Part print with two shaded views. Sizes in mm from the minimum x, y, z corner. Give positions to 0.01 mm unless a question says otherwise; leave off trailing zeros. Order: outer loops, then holes, each group sorted by start corner. A loop starts at its lowest first (then second) coordinate and runs counter-clockwise, first axis right, second up. Notation, with made-up numbers: M -21,57.25 L 2,57.25 A15 cw 2,75.25 Z; hole C 45,48.5 d2. An arc over 180 degrees is marked long. Return JSON: item names as keys, results as strings.
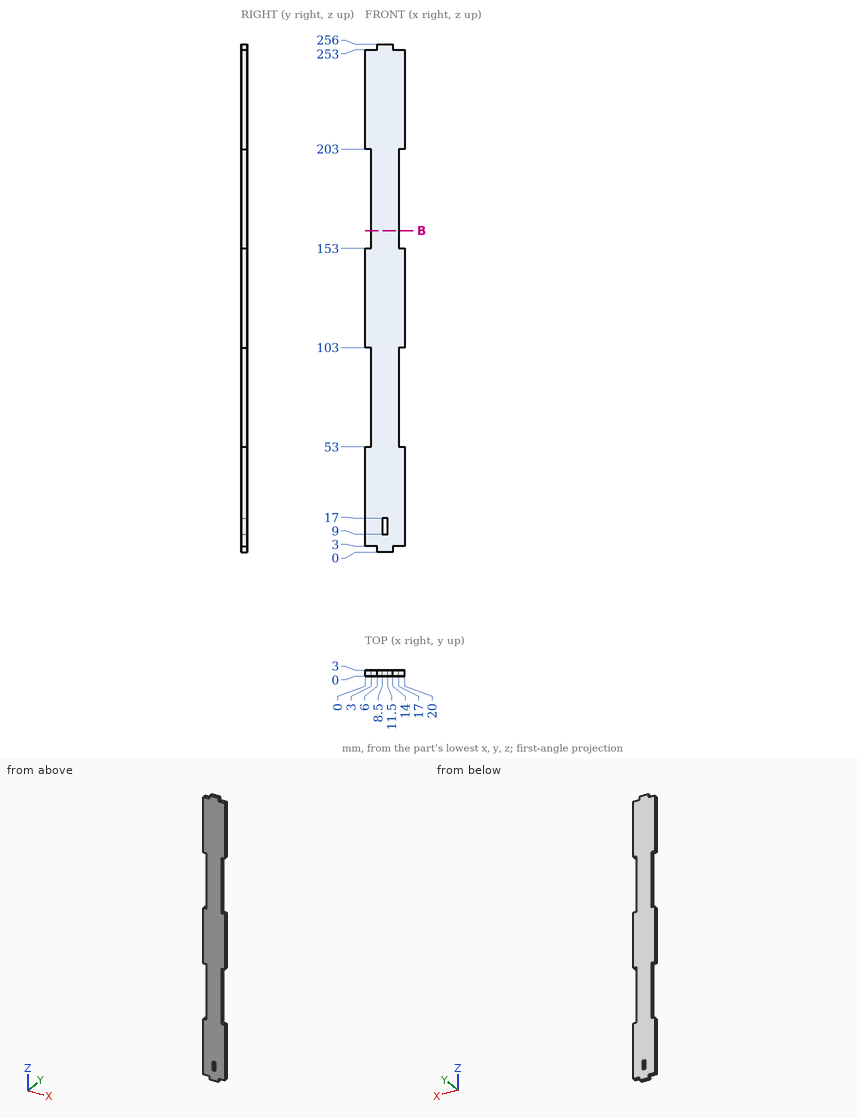
Q1. Band-saw the part on B-B (z = 162). Give the cut face in (x, y).
Established:
{"outline": "M 3,0 L 17,0 L 17,3 L 3,3 Z"}
Q2. Pin check, flat tips, straight feed: pin 1 (0.9 mm diameter, centred on x = 19, y = 1.5, fed in from -Z); pin 2 (1.5 mm diameter, centred on y = 2, z = 56.5, fed in from -X); pin 3 (1.5 mm diameter, centred on y = 2, z = 2, fed in from +X). Stop position of each tip, or through.
Established:
{"pin 1": "stops at z = 3", "pin 2": "stops at x = 3", "pin 3": "stops at x = 14"}
Q3. Probe line 1 along Z through (x, y) = (9, 2.6); line 2 along X through (y, z) = (0.7, 194); line 3 along Z through (x, y) = (3.5, 2.85). List the from-to ranges inside material, lowest first.
Established:
{"line 1": "z = 0 to 9, 17 to 256", "line 2": "x = 3 to 17", "line 3": "z = 3 to 253"}
